```python
from build123d import *

# Parameters (mm, degrees)
F0_W     = 44.0817
F0_H     = 9.3218
F0_R     = 1.905
F1_DEPTH = 0.5842
F2_W     = 44.0817
F2_H     = 9.3218
F3_DEPTH = 0.5842


with BuildPart() as f1:
    # F0 (on Top) → F1 (new body)
    with BuildSketch(Plane.XY):
        with Locations((-22.04085, 4.6609)):
            Rectangle(F0_W, F0_H)
        with Locations((-33.22955, 4.6609)):
            Circle(F0_R, mode=Mode.SUBTRACT)
        with Locations((-24.35225, 4.6609)):
            Circle(F0_R, mode=Mode.SUBTRACT)
        with Locations((-15.47495, 4.6609)):
            Circle(F0_R, mode=Mode.SUBTRACT)
        with Locations((-6.59765, 4.6609)):
            Circle(F0_R, mode=Mode.SUBTRACT)
    extrude(amount=F1_DEPTH)

    # F2 (on face) → F3 (join)
    with BuildSketch(Plane.XY.offset(0.5842)):
        with Locations((-22.04085, 4.6609)):
            Rectangle(F2_W, F2_H)
        Polygon((-27.055155, 2.931543), (-27.055155, 6.398643), (-24.35388, 7.517512), (-21.653151, 6.398869), (-21.653151, 2.931769), (-24.35388, 1.789812), align=None, mode=Mode.SUBTRACT)
        Polygon((-18.178729, 2.934289), (-18.178729, 6.401389), (-15.477454, 7.520258), (-15.47495, 7.519221), (-12.776178, 6.401393), (-12.776178, 2.934293), (-15.47495, 1.79705), align=None, mode=Mode.SUBTRACT)
        Polygon((-33.22955, 7.52475), (-30.528275, 6.407391), (-30.528275, 2.940291), (-33.22955, 1.79856), (-35.930825, 2.940291), (-35.930825, 6.407391), align=None, mode=Mode.SUBTRACT)
        Polygon((-9.259915, 3.004381), (-9.324309, 6.470883), (-6.59765, 7.52475), (-3.901778, 6.39445), (-3.901778, 2.92735), (-6.59765, 1.79705), align=None, mode=Mode.SUBTRACT)
    extrude(amount=F3_DEPTH)


solid = f1.part
```
Source: CAD feature listing. Evaluate the final solid. Frame: model axes, mm. A direction names the side the tool comes from. Round coordinates to 2 decimals unless told otherwise and drop trailing zeros. Write each loop counter-clockwise with the first axis right and the second up, starting at its lowest first coordinate (ties: lowest second). Pieces come first, ordered by that corner, then holes. Notation, with made-up numbers: M 42,78.25 L 63,78.25 A5 cw 63,83.25 Z; hole C 56.5,64.25 d1. An arc over 180 degrees is marked long. Use CSV: the item, a comma, the result in double quotes. Start each with the question number.
Q1. Line query: line 1 (X direction, y = 5, z = 0.95); line 2 (X direction, y = 4.25, z = 0.5); line 3 (Y direction, x = -15.5, z = 0.5). Output: solid intervals per line, ascending. Write a range as from..to.
Q2. Cut plane A-A on x = -16.5. Output: boundary loops of the cut face in (y, z), plus the area to 3 significant figures.
Q3. Cut plane C-C on y = 4.25. Count the separate pieces of the cut face and the enclosed holes in it, plus the area to 3 significant figures.
Q4. First-contact query: P1, Ø0.6, axis at y = 5, z = 1, coming from the +X side; P2, Ø2.5, axis at x = -7, y = 3.5, coming from the +Z side; P3, Ø3, axis at x = -6.6, y = 4.66, coming from the -Z side. Flat tips, straight axial feed; report the tip coordinate or a pass-through.
Q5. Pull-direction query (X, two-part tool) for faces 3 (the face through (-22, 7, 1.168)), 4 (the face through (-16, 7, 0.584)), 5 (the face through (-16.88, 5.95, 0.29)), 6 (the face through (0, 5, 1)); classes: +X half, -X half, draft (parallel to the pull), parting line (faces both ways), or undercut.
Q6. Access query for faces 1 (the face through (-22, 5, 0)), 2 (the face through (-25.72, 6.95, 0.87)). Directions: +Z, -Z, +X, -X, +Y, -Y. A direction counts if a zero-diameter tool reaches every point of the face in a straight line with its end or side. Return the directions, or none.
Q7. Cut plane B-B on z = 0.35. Output: boundary loops of the cut face in (x, y) (3 decimals), plus the area to 3 significant figures.
Results found:
1,line 1,"-44.08..-35.93, -30.53..-27.06, -21.65..-18.18, -12.78..-9.3, -3.9..0"
1,line 2,"-44.08..-35.09, -31.37..-26.21, -22.49..-17.34, -13.61..-8.46, -4.74..0"
1,line 3,"0..2.76, 6.57..9.32"
2,outline,"M 0,0 L 3.06,0 L 3.06,0.58 L 2.23,0.58 L 2.23,1.17 L 0,1.17 Z; M 6.27,0 L 9.32,0 L 9.32,1.17 L 7.1,1.17 L 7.1,0.58 L 6.27,0.58 Z"
2,area,"6.17 mm^2"
3,separate pieces,"5"
3,enclosed holes,"0"
3,area,"30.2 mm^2"
4,P1,"x = 0"
4,P2,"z = 0.58"
4,P3,"through"
5,face 3,"draft"
5,face 4,"undercut"
5,face 5,"undercut"
5,face 6,"+X half"
6,face 1,"-Z, +X, -X, +Y, -Y"
6,face 2,"+Z"
7,outline,"M -44.082,0 L 0,0 L 0,9.322 L -44.082,9.322 Z; hole C -33.23,4.661 d3.81; hole C -24.352,4.661 d3.81; hole C -15.475,4.661 d3.81; hole C -6.598,4.661 d3.81"
7,area,"365 mm^2"
